Can you work these out from the drawing? Everything is in mm from the part's minimum corner. A direction names the side the tool comes from. Round coordinates to 2 decimals unless told otherwise and drop trailing zeros. Loops run counter-clockwise (first coordinate to the right, second up) from the corner with the lowest first, then second, coordinate; pieces in that order, holes last. Notation, with made-up numbers: M 61.5,58 L 99.5,58 A18 cw 99.5,73 Z; hole C 4,87.5 d6. An arc over 180 degrees is marked long. Answer in a Markdown table with one row per item.
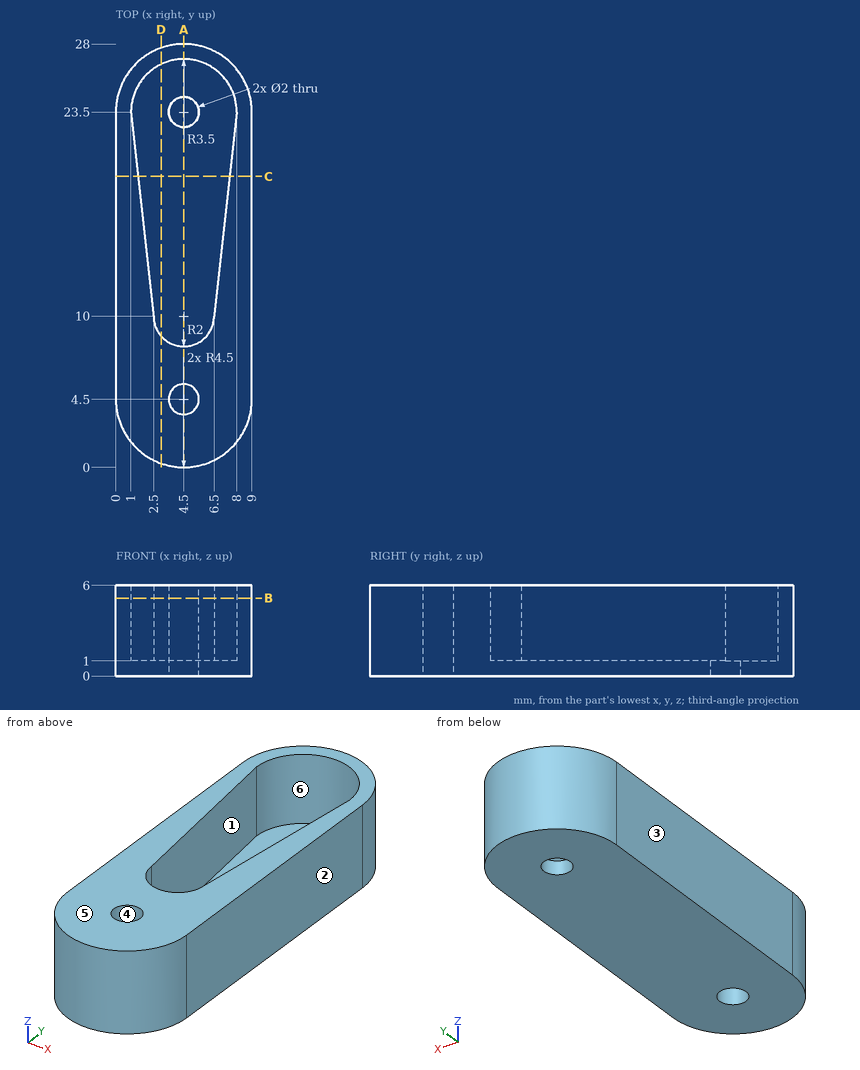
1) I want a section at B-B, the plane z = 5.15. Please give me the cut outline in (x, y), plus the area to 3 significant figures.
Computed:
| item | result |
|---|---|
| outline | M 0,4.5 A4.5 ccw 9,4.5 L 9,23.5 A4.5 ccw 0,23.5 Z; hole M 1,23.5 L 2.5,10 A2 ccw 6.5,10 L 8,23.5 A3.5 ccw Z; hole C 4.5,4.5 d2 |
| area | 132 mm² |
2) I want a section at D-D, the plane x = 3. Please give me the cut outline in (y, z).
Computed:
| item | result |
|---|---|
| outline | M 0.26,0 L 27.74,0 L 27.74,6 L 26.66,6 L 26.66,1 L 8.68,1 L 8.68,6 L 0.26,6 Z |
3) I want a section at A-A, the plane x = 4.5. Please give me the cut outline in (y, z), plus the area to 3 significant figures.
Computed:
| item | result |
|---|---|
| outline | M 0,0 L 3.5,0 L 3.5,6 L 0,6 Z; M 5.5,0 L 22.5,0 L 22.5,1 L 8,1 L 8,6 L 5.5,6 Z; M 24.5,0 L 28,0 L 28,6 L 27,6 L 27,1 L 24.5,1 Z |
| area | 59.0 mm² |
4) I want a section at C-C, the plane y = 19.25. Please give me the cut outline in (x, z).
Computed:
| item | result |
|---|---|
| outline | M 0,0 L 9,0 L 9,6 L 7.53,6 L 7.53,1 L 1.47,1 L 1.47,6 L 0,6 Z |
5) If we mould it in two halves opening along X, with no side actions, what happens to the marked faces 3, 4, 5 and 6? For each: released by +X, released by -X, zero draft, split by the parting line, or undercut.
Computed:
| item | result |
|---|---|
| face 3 | released by -X |
| face 4 | undercut |
| face 5 | zero draft |
| face 6 | undercut |
6) Which directions (+Z, -Z, +X, -X, +Y, -Y) give clear straight access to the entire face, cutting with the end or side of a thin tool? Please do the marked faces 1 and 2.
Computed:
| item | result |
|---|---|
| face 1 | +Z |
| face 2 | +Z, -Z, +X, +Y, -Y |
7) Will these pins go through, and if not, where does the flat tip stop? P1, Ø1, axis at x = 2.5, z = 1.5, coming from the -Y side; P2, Ø2, axis at x = 5.5, z = 1.5, coming from the -Y side; P3, Ø2, axis at x = 4.5, y = 12, coming from the +Z side.
Computed:
| item | result |
|---|---|
| P1 | stops at y = 0.26 |
| P2 | stops at y = 0 |
| P3 | stops at z = 1 |
8) I need wall thicknesses on line 1 (Y direction, x = 4.5, z = 4); line 2 (Y direction, x = 4.5, z = 0.65); line 3 (X direction, y = 23.5, z = 0.7). Which ranges of each line are inside material? Lowest first, please.
Computed:
| item | result |
|---|---|
| line 1 | y = 0 to 3.5, 5.5 to 8, 27 to 28 |
| line 2 | y = 0 to 3.5, 5.5 to 22.5, 24.5 to 28 |
| line 3 | x = 0 to 3.5, 5.5 to 9 |
